```python
from build123d import *

# Parameters (mm, degrees)
SKETCH2_W                  = 15
SKETCH2_H                  = 17.79
SKETCH2_R                  = 1.5
BASE_FLANGE1_DEPTH         = 2
SKETCHED_BEND6_OUTLINE_W   = 2
SKETCHED_BEND6_OUTLINE_H   = 17.79
SKETCHED_BEND6_DEPTH       = 5.5
SKETCHED_START             = 5.74315
SKETCHED_BEND6_2_OUTLINE_W = 8.49
SKETCHED_BEND6_2_OUTLINE_H = 17.79
SKETCHED_BEND6_2_OUTLINE_R = 1.5
SKETCHED_BEND6_2_DEPTH     = 1.75685
SKETCHED_START_2           = 5.5
SKETCHED_BEND6_3_OUTLINE_W = 8.49
SKETCHED_BEND6_3_OUTLINE_H = 17.79
SKETCHED_BEND6_3_OUTLINE_R = 1.5
SKETCHED_BEND6_3_DEPTH     = 2.5
SKETCHED_START_3           = -17.79
SKETCHED_BEND6_4_DEPTH     = 17.79
FILLET1_R                  = 0.5


with BuildPart() as part:
    # Base-Flange1: sheet metal written as solids
    # Sketch2 → Base-Flange1 (new body)
    with BuildSketch(Plane(origin=(0, 0, 0), x_dir=(1, 0, 0), z_dir=(0, 1, 0))):
        with Locations((7.5, 8.895)):
            Rectangle(SKETCH2_W, SKETCH2_H)
        with Locations(Location((11.51, 14.145, 0), (0, 0, 270))):
            Circle(SKETCH2_R, mode=Mode.SUBTRACT)
        with Locations(Location((11.51, 3.645, 0), (0, 0, 270))):
            Circle(SKETCH2_R, mode=Mode.SUBTRACT)
        with Locations(Location((3.49, 3.645, 0), (0, 0, 270))):
            Circle(SKETCH2_R, mode=Mode.SUBTRACT)
        with Locations(Location((3.49, 14.145, 0), (0, 0, 270))):
            Circle(SKETCH2_R, mode=Mode.SUBTRACT)
    extrude(amount=-BASE_FLANGE1_DEPTH)

    # Sketched Bend6: read off the stored shape, not the designer's step
    # Sketched Bend6 outline → Sketched Bend6 (cut)
    with BuildSketch(Plane.YZ):
        with Locations((-1, -8.895)):
            Rectangle(SKETCHED_BEND6_OUTLINE_W, SKETCHED_BEND6_OUTLINE_H)
    extrude(amount=SKETCHED_BEND6_DEPTH, mode=Mode.SUBTRACT)

    # Sketched Bend6 2 outline → Sketched Bend6 2 (add)
    with BuildSketch(Plane.YZ.offset(SKETCHED_START)):
        with Locations((4.245, -8.895)):
            Rectangle(SKETCHED_BEND6_2_OUTLINE_W, SKETCHED_BEND6_2_OUTLINE_H)
        with Locations((5, -14.145)):
            Circle(SKETCHED_BEND6_2_OUTLINE_R, mode=Mode.SUBTRACT)
        with Locations((5, -3.645)):
            Circle(SKETCHED_BEND6_2_OUTLINE_R, mode=Mode.SUBTRACT)
    extrude(amount=SKETCHED_BEND6_2_DEPTH)

    # Sketched Bend6 3 outline → Sketched Bend6 3 (add)
    with BuildSketch(Plane.YZ.offset(SKETCHED_START_2)):
        with Locations((4.245, -8.895)):
            Rectangle(SKETCHED_BEND6_3_OUTLINE_W, SKETCHED_BEND6_3_OUTLINE_H)
        with Locations((5, -14.145)):
            Circle(SKETCHED_BEND6_3_OUTLINE_R, mode=Mode.SUBTRACT)
        with Locations((5, -3.645)):
            Circle(SKETCHED_BEND6_3_OUTLINE_R, mode=Mode.SUBTRACT)
    extrude(amount=SKETCHED_BEND6_3_DEPTH)

    # Sketched Bend6 4 outline → Sketched Bend6 4 (cut)
    with BuildSketch(Plane.XY.offset(SKETCHED_START_3)):
        with BuildLine():
            Line((8, 8.49), (7.5, 8.49))
            Line((7.5, 8.49), (7.5, 0.5))
            ThreePointArc((7.5, 0.5), (7.646446609, 0.146446609), (8, 0))
            Line((8, 0), (8, 8.49))
        make_face()
        with BuildLine():
            ThreePointArc((8, -2), (6.232233047, -1.267766953), (5.5, 0.5))
            Line((5.5, 0.5), (5.5, -2))
            Line((5.5, -2), (8, -2))
        make_face()
    extrude(amount=SKETCHED_BEND6_4_DEPTH, mode=Mode.SUBTRACT)

    # Fillet1
    fillet1_edges = [part.edges().sort_by_distance(p)[0] for p in [
        (15, -1, -17.79),
        (15, -1, 0),
        (6.5, 8.49, -17.79),
        (6.5, 8.49, 0),
    ]]
    fillet(fillet1_edges, radius=FILLET1_R)


solid = part.part
```
The listing builds one solid part. Answer for the finished solid, in the listing's coordinates (mm). A direction names the side the tool comes from. Round coordinates to 2 decimals unless told otherwise and drop trailing zeros. Loops run counter-clockwise (first coordinate to the right, second up) from the corner with the lowest first, then second, coordinate; pieces in that order, holes last.
Q1. For a pull along Z with two mould halves and no side action, classify faces 3 (the face through (10.046, -0.986, -3.97)), 4 (the face through (11, 0, -9)), 5 (the face through (7, 2, -17.79)) as released by +Z, released by -Z, zero draft, split by the parting line, or undercut.
Q2. Section D-D, the plane y = 2 is taken. Determine the outline of the cut face in (x, z), then the cut area to 3 significant figures.
Q3. Section C-C, the plane z = -10.25 is taken. Determine the outline of the cut face in (x, y), then the cut area to 3 significant figures.
Q4. Which of the six approach directions +Z, -Z, +X, -X, +Y, -Y give full straight-line access (tool end or side, diameter ignored) to faces 1 (the face through (6.486, 5.806, -12.88)), 2 (the face through (7.5, 5, -9))?
Q5. Section B-B, the plane x = 11.51 is taken. Determine the outline of the cut face in (y, z) (3 decimals).
Q6. Find the intervals of material crossed by line 1 (Z direction, x = 6.05, y = 5) (3 decimals); line 2 (Z direction, x = 10.25, y = -0.75); line 3 (X direction, y = 2, z = -16.25), in increasing order.
Q7. Given pin 1 Ø3.5 at (x, z) = (11.51, -14.145) entering from -Y; pin 2 Ø3.5 at (y, z) = (5, -14.145) entering from +X; pin 3 Ø1.5 at (x, z) = (11, -13.5) entering from +Y, each flat-ended and moving along its own axis, determine where each tip first touches the part or whether it passes through.
Q8. Section A-A, the plane y = 5 is taken. Determine the outline of the cut face in (x, z) (3 decimals).
Completed:
1. face 3: undercut
1. face 4: zero draft
1. face 5: released by -Z
2. outline: (5.5, -17.79) - (7.5, -17.79) - (7.5, 0) - (5.5, 0) - close
2. area: 35.6 mm2
3. outline: (5.5, 0.5) arc R2.5 ccw to (8, -2) - (15, -2) - (15, 0) - (8, 0) arc R0.5 cw to (7.5, 0.5) - (7.5, 8.49) - (5.5, 8.49) - close
3. area: 34.7 mm2
4. face 1: +X, -X
4. face 2: +Z, -Z, +X, +Y
5. outline: (-2, -17.79) - (0, -17.79) - (0, -15.645) - (-2, -15.645) - close; (-2, -12.645) - (0, -12.645) - (0, -5.145) - (-2, -5.145) - close; (-2, -2.145) - (0, -2.145) - (0, 0) - (-2, 0) - close
6. line 1: z = -17.79 to -15.645, -12.645 to -5.145, -2.145 to 0
6. line 2: z = -17.79 to -14.96, -13.33 to -4.46, -2.83 to 0
6. line 3: x = 5.5 to 7.5
7. pin 1: stops at y = -2
7. pin 2: stops at x = 7.5
7. pin 3: stops at y = 0
8. outline: (5.5, -17.79) - (7.5, -17.79) - (7.5, -15.645) - (5.5, -15.645) - close; (5.5, -12.645) - (7.5, -12.645) - (7.5, -5.145) - (5.5, -5.145) - close; (5.5, -2.145) - (7.5, -2.145) - (7.5, 0) - (5.5, 0) - close
